For this review, take the finished solid that the model builds, in its own axes (mm). Face numbers are marked on the shaded views. A direction names the side the tool comes from. Round coordinates to 2 decimals unless told otherwise and drop trailing zeros. Order: outer loops, then holes, each group sorted by start corner. A loop starts at its lowest first (then second) coordinate and runs counter-clockwise, first axis right, second up. Notation, with made-up numbers: (71, 89) - (123, 89) arc R23 cw to (123, 108) - close; hole circle Ø9 at (30.25, 69.25). An arc over 180 degrees is marked (long way). Write each question's results on one line, items separated by ' | '. Start each with the question number.
(1) For the marked faces 1 and 2, list the 3-axis set-ups (+Z, -Z, +X, -X, +Y, -Y) from which the entire face can be reached by the end or side of a thin tool; tool diameter is ignored.
(2) For L1, parallel to Y at x = -16, z = 0; L2, parallel to Y at x = 48, z = 35; L3, parallel to X at y = -17, z = 34.5, list the stretches that pass through material, from the lowest coordinate up. Write a range as from..to.
(3) Take a section at B-B, the plane z = -7. Give the boundary of the cut face in (x, y), plus the area to 3 significant figures.
(4) Take a section at A-A, the plane x = -7. Give the boundary of the cut face in (y, z).
(5) Insertion check: pin 1 Ø2 at (y, z) = (-15, -16) entering from +X; pin 2 Ø0.8 at (x, y) = (-12, -18) entering from -Z. Each pin has a flat end and moves straight along its axis. Give the tip position at first contact, or say it passes through.
(6) Take a section at D-D, the plane x = 64. Give the boundary of the cut face in (y, z), plus the area to 3 significant figures.
(7) Take a section at C-C, the plane z = -37. Give the boundary of the cut face in (x, y), plus the area to 3 significant figures.
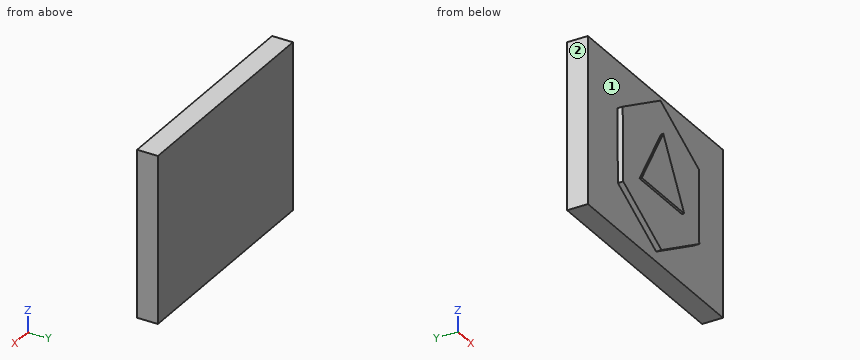
```python
from build123d import *

# Parameters (mm, degrees)
F0_W     = 152.150162
F0_H     = 111.926563
F1_DEPTH = 13.97
F3_DEPTH = 3.556
F5_DEPTH = 1.524


with BuildPart() as f1:
    # F0 (on Front) → F1 (new body)
    with BuildSketch(Plane.XZ):
        with Locations((-0.291478, -0.145737)):
            Rectangle(F0_W, F0_H)
    extrude(amount=F1_DEPTH)

    # F2 (on face) → F3 (join)
    with BuildSketch(Plane.XZ.offset(13.97)):
        Polygon((-0.572803, 49.492897), (-43.148508, 24.250387), (-42.575705, -25.242511), (0.572803, -49.492897), (43.148508, -24.250387), (42.575705, 25.242511), align=None)
    extrude(amount=F3_DEPTH)

    # F4 (on face) → F5 (join)
    with BuildSketch(Plane.XZ.offset(17.526)):
        Polygon((23.607507, -14.136557), (0, 27.25295), (-24.19246, -14.136557), align=None)
    extrude(amount=F5_DEPTH)


solid = f1.part
```
Results below:
1) face 1: -Y | face 2: +Z, -Z, -X, +Y, -Y
2) L1: y = -17.53..0 | L2: y = -13.97..0 | L3: x = -25.86..26.1
3) outline: (-76.37, -13.97) - (-42.79, -13.97) - (-42.79, -17.53) - (-20.02, -17.53) - (-20.02, -19.05) - (19.54, -19.05) - (19.54, -17.53) - (42.95, -17.53) - (42.95, -13.97) - (75.78, -13.97) - (75.78, 0) - (-76.37, 0) - close | area: 2,490 mm^2
4) outline: (-19.05, -14.14) - (-17.53, -14.14) - (-17.53, -45.24) - (-13.97, -45.24) - (-13.97, -56.11) - (0, -56.11) - (0, 55.82) - (-13.97, 55.82) - (-13.97, 45.68) - (-17.53, 45.68) - (-17.53, 15.28) - (-19.05, 15.28) - close
5) pin 1: stops at x = 43.06 | pin 2: stops at z = -14.14
6) outline: (-13.97, -56.11) - (0, -56.11) - (0, 55.82) - (-13.97, 55.82) - close | area: 1,560 mm^2
7) outline: (-76.37, -13.97) - (-21.66, -13.97) - (-21.66, -17.53) - (21.64, -17.53) - (21.64, -13.97) - (75.78, -13.97) - (75.78, 0) - (-76.37, 0) - close | area: 2,280 mm^2
